from build123d import *

# Parameters (mm, degrees)
SKETCH1_W           = 133
SKETCH1_H           = 110
BOSS_EXTRUDE1_DEPTH = 3
SKETCH2_W           = 50
SKETCH2_H           = 18
SKETCH2_W_2         = 41
SKETCH2_H_2         = 15
SKETCH2_W_3         = 31
BOSS_EXTRUDE2_DEPTH = 3
CUT_EXTRUDE1_REACH  = 8
SKETCH3_R           = 12.5
SKETCH3_R_2         = 15.25
SKETCH4_R           = 16.375
CUT_EXTRUDE2_DEPTH  = 1


with BuildPart() as part:
    # Sketch1 → Boss-Extrude1 (new body)
    with BuildSketch(Plane(origin=(0, 0, 0), x_dir=(1, 0, 0), z_dir=(0, 1, 0))):
        with Locations((66.5, 55)):
            Rectangle(SKETCH1_W, SKETCH1_H)
    extrude(amount=BOSS_EXTRUDE1_DEPTH)

    # Sketch2 → Boss-Extrude2 (add)
    with BuildSketch(Plane.XZ):
        with Locations((25, -109)):
            Rectangle(SKETCH2_W, SKETCH2_H)
        with Locations((112.5, -2.5)):
            Rectangle(SKETCH2_W_2, SKETCH2_H_2)
        with Locations((23.5, -2.5)):
            Rectangle(SKETCH2_W_3, SKETCH2_H_2)
    extrude(amount=BOSS_EXTRUDE2_DEPTH)

    # Sketch3 → Cut-Extrude1 (cut, up to next)
    with BuildSketch(Plane(origin=(0, 3, 0), x_dir=(1, 0, 0), z_dir=(0, 1, 0)), mode=Mode.PRIVATE) as cut_extrude1_sk1:
        with Locations((65.5, 42.75)):
            Circle(SKETCH3_R)
    cut_extrude1_tool1 = extrude(cut_extrude1_sk1.sketch, amount=-CUT_EXTRUDE1_REACH, mode=Mode.PRIVATE) & part.part
    add(cut_extrude1_tool1.solids().sort_by_distance((65.5, 3, -42.75))[0], mode=Mode.SUBTRACT)
    # Sketch3 → Cut-Extrude1 (cut, up to next)
    with BuildSketch(Plane(origin=(0, 3, 0), x_dir=(1, 0, 0), z_dir=(0, 1, 0)), mode=Mode.PRIVATE) as cut_extrude1_sk2:
        with Locations((128.5, 28.75)):
            Circle(SKETCH3_R_2)
    cut_extrude1_tool2 = extrude(cut_extrude1_sk2.sketch, amount=-CUT_EXTRUDE1_REACH, mode=Mode.PRIVATE) & part.part
    add(cut_extrude1_tool2.solids().sort_by_distance((128.5, 3, -28.75))[0], mode=Mode.SUBTRACT)
    # Sketch3 → Cut-Extrude1 (cut, up to next)
    with BuildSketch(Plane(origin=(0, 3, 0), x_dir=(1, 0, 0), z_dir=(0, 1, 0)), mode=Mode.PRIVATE) as cut_extrude1_sk3:
        with Locations((135.5, 67.25)):
            Circle(SKETCH3_R_2)
    cut_extrude1_tool3 = extrude(cut_extrude1_sk3.sketch, amount=-CUT_EXTRUDE1_REACH, mode=Mode.PRIVATE) & part.part
    add(cut_extrude1_tool3.solids().sort_by_distance((135.5, 3, -67.25))[0], mode=Mode.SUBTRACT)

    # Sketch4 → Cut-Extrude2 (cut)
    with BuildSketch(Plane.XZ):
        with Locations((128.5, -28.75)):
            Circle(SKETCH4_R)
        with Locations((135.5, -67.25)):
            Circle(SKETCH4_R)
    extrude(amount=-CUT_EXTRUDE2_DEPTH, mode=Mode.SUBTRACT)


solid = part.part
Build history of the part. All positions in model axes, mm. A direction names the side the tool comes from. Round coordinates to 2 decimals unless told otherwise and drop trailing zeros. Loops run counter-clockwise (first coordinate to the right, second up) from the corner with the lowest first, then second, coordinate; pieces in that order, holes last. Notation, with made-up numbers: (-37.5, 53) -> (6.5, 53) arc R22 ccw to (6.5, 61) -> close; hole circle Ø3 at (5.25, -33). An arc over 180 degrees is marked (long way). Use CSV: the item, a comma, the result in double quotes. Start each with the question number.
Q1. Mould opens along Z. For faces 1 (the face through (92, -1, -3)), 2 (the face through (113.255, 2.014, -29.149)), 3 (the face through (112, -1, -10)), 4 (the face through (119.13, 0.49, -66.93)) say: +Z half, -Z half, draft (parallel to the pull), parting line (faces both ways), or undercut.
Q2. Flat gauge pins, fed straight in: pin 1 Ø20 at (x, z) = (65.5, -42.75) entering from +Y; pin 2 Ø0.9 at (x, y) = (111, -2) entering from -Z; pin 3 Ø0.9 at (y, z) = (-1.5, -3) entering from -X; pin 4 Ø3.5 at (x, y) = (74, 1) entering from -Z. Where does each tip first touch, or does it go through?
Q3. Saw through at A-A on x = 65.5. Give the cut face in (y, z), and give its area (3 significant figures).
Q4. Which spindle directions (+Z, -Z, +X, -X, +Y, -Y) get a long thin tool onto all of the face, cutting with end or side? Do faces 5 (the face through (8, -1, -3)), 6 (the face through (23, 0, 3)), 7 (the face through (25, -1, -100)). Say none if no direction does.
Q5. Saw through at C-C on x = 128.5. Give the cut face in (y, z) (3 decimals).
Q6. Drill centre lines: L1, parallel to Z at x = 128.5, y = 1.55; L2, parallel to X at y = 1.45, z = -28.75; L3, parallel to X at y = 1.05, z = -47. Where is each one in solid material? Low to high.
Q7. Saw through at B-B on z = -37.5. Give the cut face in (x, y).
Q8. Saw through at D-D on x = 94. Give the cut face in (y, z).
Solutions:
1,face 1,"draft"
1,face 2,"undercut"
1,face 3,"-Z half"
1,face 4,"undercut"
2,pin 1,"passes through"
2,pin 2,"stops at z = -10"
2,pin 3,"stops at x = 8"
2,pin 4,"stops at z = -110"
3,outline,"(0, -110) -> (3, -110) -> (3, -55.25) -> (0, -55.25) -> close; (0, -30.25) -> (3, -30.25) -> (3, 0) -> (0, 0) -> close"
3,area,"255 mm^2"
4,face 5,"+Z, -X, -Y"
4,face 6,"+Z, +X, -X, +Y"
4,face 7,"+X, -X, -Y"
5,outline,"(-3, -10) -> (0, -10) -> (0, -12.375) -> (1, -12.375) -> (1, -13.5) -> (3, -13.5) -> (3, 0) -> (0, 0) -> (0, 5) -> (-3, 5) -> close; (0, -110) -> (3, -110) -> (3, -80.799) -> (1, -80.799) -> (1, -82.053) -> (0, -82.053) -> close; (0, -52.447) -> (1, -52.447) -> (1, -53.701) -> (3, -53.701) -> (3, -44) -> (1, -44) -> (1, -45.125) -> (0, -45.125) -> close"
6,L1,"z = -110 to -80.8, -53.7 to -44, -13.5 to 0"
6,L2,"x = 0 to 113.25"
6,L3,"x = 0 to 53.74, 77.26 to 133"
7,outline,"(0, 0) -> (54.16, 0) -> (54.16, 3) -> (0, 3) -> close; (76.84, 0) -> (114.66, 0) -> (114.66, 1) -> (116.01, 1) -> (116.01, 3) -> (76.84, 3) -> close"
8,outline,"(-3, -10) -> (0, -10) -> (0, -110) -> (3, -110) -> (3, 0) -> (0, 0) -> (0, 5) -> (-3, 5) -> close"
